Can you work these out from the model? Positions are in its coordinate system, mm. A direction names the side the tool comes from. Round coordinates to 2 decimals unless told otherwise and drop trailing zeros. Write each loop counter-clockwise with the first axis right and the second up, starting at its lowest first coordinate (ties: lowest second). Pieces come first, ordered by that corner, then holes. Notation, with made-up numbers: (84, 50.25) - (112, 50.25) arc R11 ccw to (112, 68.25) - close; hole circle Ø10 at (56.25, 12.5). An arc over 180 degrees is marked (long way). One line per item, written item: value. Start each with the question number.
(1) On a 3-axis mill with a long thin cutter (end or side, diameter ignored), from which of +Z, -Z, +X, -X, +Y, -Y can I reach the whole of each face in a straight line? I mean faces 1 (the face through (18, -3, 6)), 2 (the face through (19.53, -3.45, 5.24)), 3 (the face through (10.597, 4.801, 1.479)). Say none if no direction works.
(2) I want a section at D-D on y = 4.5. List the corners of the cut face in (x, z) for me, plus the area to 3 significant figures.
(3) I want a section at A-A on z = 1.5. List the corners of the cut face in (x, y) for me (3 decimals).
(4) If I drill on L1, parallel to Z at x = 25.5, y = -1.5; L2, parallel to Y at x = 10, z = 2; L3, parallel to X at y = -3.6, z = 4.5, over which ranges is the centre line in solid material (lowest first)? Write a range as from..to.
(5) I want a section at B-B on y = -1.75. List the corners of the cut face in (x, z) for me.
(6) I want a section at C-C on x = 27. List the corners of the cut face in (y, z) for me.
(7) I'm going to push flat-ended pins straight in: pin 1 Ø1.5 at (x, z) = (28, 2) entering from -Y; pin 2 Ø1.8 at (x, z) = (19.84, 4.5) entering from -Y; pin 3 Ø2 at (x, y) = (26.5, -1.5) entering from +Z. Where does each tip first touch, or does it pass through?
(8) Thinking about a two-plate mould opening in Y: for faces 4 (the face through (10.571, -4.765, 1.479)), 5 (the face through (21.46, 2.55, 3.04)), 6 (the face through (15.843, 0.249, 4.479)), 7 (the face through (31, 0, 3)), which applies, +Y half, -Y half, draft (parallel to the pull), parting line (faces both ways), or undercut?
from build123d import *

# Parameters (mm, degrees)
BOSS_EXTRUDE1_DEPTH     = 3
SKETCH8_R               = 4
BOSS_EXTRUDE4_DEPTH     = 3
CUT_EXTRUDE5_REACH      = 42.577
SKETCH9_R               = 3.025
CUT_EXTRUDE6_REACH      = 42.577
CUT_EXTRUDE6_END_RADIUS = 4
SKETCH10_R              = 0.8


with BuildPart() as part:
    # Sketch3 → Boss-Extrude1 (new body)
    with BuildSketch(Plane.XY):
        Polygon((0, 0), (11.497632607, 6.066666667), (9.670080369, 3.5), (39.670080369, 3.5), (39.670080369, -3.5), (9.670080369, -3.5), (11.497632607, -6.066666667), align=None)
    extrude(amount=BOSS_EXTRUDE1_DEPTH)

    # Sketch8 → Boss-Extrude4 (add)
    with BuildSketch(Plane.XY.offset(3)):
        with Locations(Location((19.835040185, 0, 0), (0, 0, 118.955024372))):
            Circle(SKETCH8_R)
    extrude(amount=BOSS_EXTRUDE4_DEPTH)

    # Sketch9 → Cut-Extrude5 (cut, up to next)
    with BuildSketch(Plane.XY.offset(6), mode=Mode.PRIVATE) as cut_extrude5_sk1:
        with Locations((19.835040185, 0)):
            Circle(SKETCH9_R)
    cut_extrude5_tool1 = extrude(cut_extrude5_sk1.sketch, amount=-CUT_EXTRUDE5_REACH, mode=Mode.PRIVATE) & part.part
    add(cut_extrude5_tool1.solids().sort_by_distance((19.83504, 0, 6))[0], mode=Mode.SUBTRACT)

    # Cut-Extrude6: up to this cylinder (the profile starts inside it)
    cut_extrude6_end = Plane(origin=(19.835040185, 0, 4.5), z_dir=(0, 0, -1)) * Cylinder(CUT_EXTRUDE6_END_RADIUS, 94.154, mode=Mode.PRIVATE)
    # Sketch10 → Cut-Extrude6 (cut, up to the surface)
    with BuildSketch(Plane(origin=(0, 0, 0), x_dir=(1, 0, 0), z_dir=(0, 1, 0)), mode=Mode.PRIVATE) as cut_extrude6_sk1:
        with Locations(Location((19.835040185, -4.5, 0), (0, 0, 270))):
            Circle(SKETCH10_R)
    cut_extrude6_tool1 = extrude(cut_extrude6_sk1.sketch, amount=-CUT_EXTRUDE6_REACH, mode=Mode.PRIVATE) & cut_extrude6_end
    add(cut_extrude6_tool1.solids().sort_by_distance((19.83504, 0, 4.5))[0], mode=Mode.SUBTRACT)


solid = part.part
Established:
1. face 1: +Z, +X, -X, +Y, -Y
1. face 2: -Y
1. face 3: +Z, -Z, +X
2. outline: (8.53, 0) - (10.38, 0) - (10.38, 3) - (8.53, 3) - close
2. area: 5.56 mm2
3. outline: (0, 0) - (11.498, -6.067) - (9.67, -3.5) - (39.67, -3.5) - (39.67, 3.5) - (9.67, 3.5) - (11.498, 6.067) - close; hole circle Ø6.05 at (19.835, 0)
4. L1: 0..3
4. L2: -5.28..-3.96, -3.5..3.5, 3.96..5.28
4. L3: 18.09..19.04, 20.64..21.58
5. outline: (3.32, 0) - (17.37, 0) - (17.37, 6) - (16.24, 6) - (16.24, 3) - (3.32, 3) - close; (22.3, 0) - (39.67, 0) - (39.67, 3) - (23.43, 3) - (23.43, 6) - (22.3, 6) - close
6. outline: (-3.5, 0) - (3.5, 0) - (3.5, 3) - (-3.5, 3) - close
7. pin 1: y = -3.5
7. pin 2: y = -4
7. pin 3: z = 3
8. face 4: undercut
8. face 5: undercut
8. face 6: parting line
8. face 7: draft
